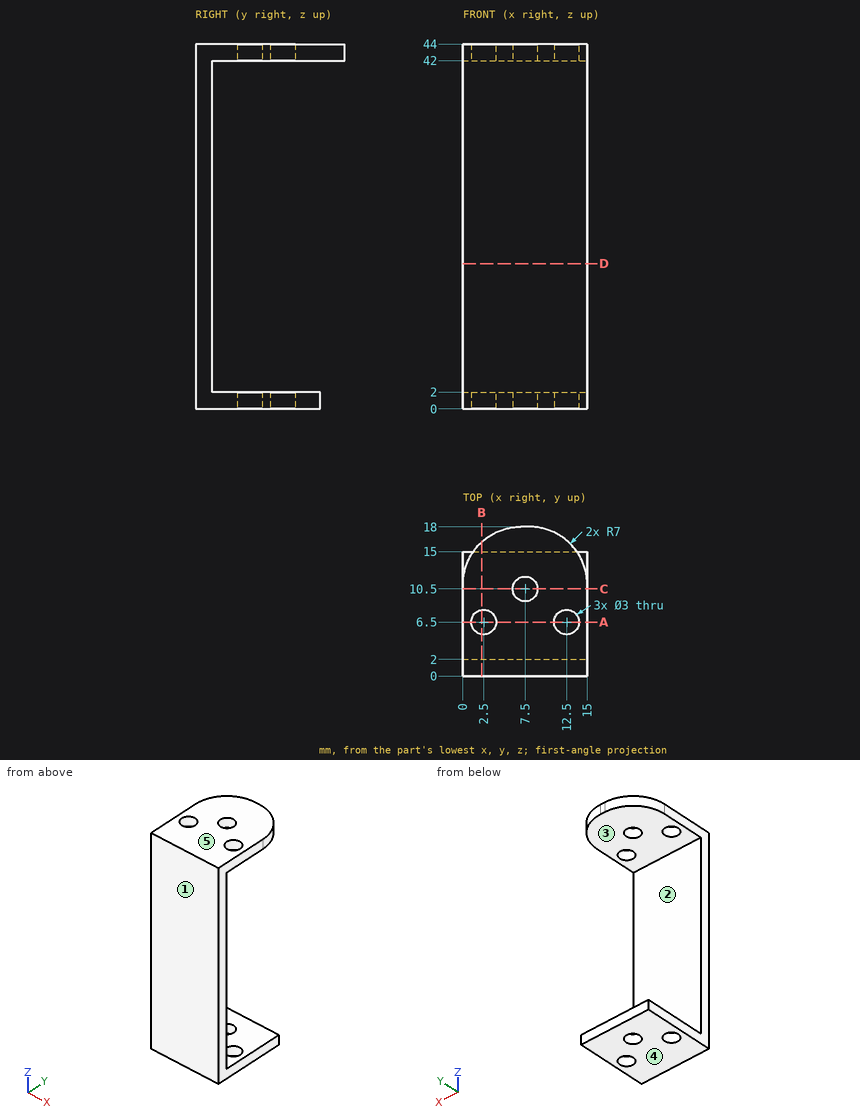
Part print with two shaded views. Sizes in mm from the minimum x, y, z corner. A direction names the side the tool comes from. Give positions to 0.01 mm unless a question says otherwise; leave off trailing zeros. Order: outer loops, then holes, each group sorted by start corner. A loop starts at its lowest first (then second) coordinate and runs counter-clockwise, first axis right, second up.
(1) Mould opens along Z. For the marked faces 3, 4 and 5 say: released by +Z, released by -Z, zero draft, split by the parting line, or undercut.
(2) Tool access for the marked faces 1 and 2: list every direction of +Z, -Z, +X, -X, +Y, -Y with a clear straight run to the whole face (end or side of a thin tool).
(3) Flat gauge pins, fed straight in: pin 1 (6 mm diameter, centred on x = 2, z = 31.5, fed in from -Y); pin 2 (2.5 mm diameter, centred on x = 7.5, y = 10.5, fed in from +Z); pin 3 (1.6 mm diameter, centred on x = 8, z = 1, fed in from +Y). Where does each tip first touch, or does it go through?
(4) Saw through at D-D, the plane z = 17.5. Give the cut face in (x, y).
(5) Saw through at B-B, the plane x = 2.25. Give the cut face in (y, z).
(6) Drill centre lines: L1, parallel to X at y = 6.5, z = 1.6; L2, parallel to Y at x = 12.5, z = 1.05; L3, parallel to Z at x = 2, y = 13. Where is each one in solid material? Low to high.
(7) Saw through at A-A, the plane y = 6.5. Give the cut face in (x, z).
(8) Saw through at C-C, the plane y = 10.5. Give the cut face in (x, z).
Results found:
1. face 3: undercut
1. face 4: released by -Z
1. face 5: released by +Z
2. face 1: +Z, -Z, +X, -X, -Y
2. face 2: +X, -X, +Y
3. pin 1: stops at y = 0
3. pin 2: passes through
3. pin 3: stops at y = 15
4. outline: (0, 0) - (15, 0) - (15, 2) - (0, 2) - close
5. outline: (0, 0) - (5.02, 0) - (5.02, 2) - (2, 2) - (2, 42) - (5.02, 42) - (5.02, 44) - (0, 44) - close; (7.98, 0) - (15, 0) - (15, 2) - (7.98, 2) - close; (7.98, 42) - (16.14, 42) - (16.14, 44) - (7.98, 44) - close
6. L1: x = 0 to 1, 4 to 11, 14 to 15
6. L2: y = 0 to 5, 8 to 15
6. L3: z = 0 to 2, 42 to 44
7. outline: (0, 0) - (1, 0) - (1, 2) - (0, 2) - close; (0, 42) - (1, 42) - (1, 44) - (0, 44) - close; (4, 0) - (11, 0) - (11, 2) - (4, 2) - close; (4, 42) - (11, 42) - (11, 44) - (4, 44) - close; (14, 0) - (15, 0) - (15, 2) - (14, 2) - close; (14, 42) - (15, 42) - (15, 44) - (14, 44) - close
8. outline: (0, 0) - (6, 0) - (6, 2) - (0, 2) - close; (0, 42) - (6, 42) - (6, 44) - (0, 44) - close; (9, 0) - (15, 0) - (15, 2) - (9, 2) - close; (9, 42) - (15, 42) - (15, 44) - (9, 44) - close
